Source: CAD feature listing. Evaluate the final solid. Frame: model axes, mm. A direction names the side the tool comes from. Give positions to 0.01 mm unless a question says otherwise; leave off trailing zeros. Order: outer loops, then holes, each group sorted by start corner. A loop starts at its lowest first (then second) coordinate and runs counter-clockwise, first axis right, second up. Notation, with made-up numbers: (37, 32) -> (94, 32) arc R18 ccw to (94, 61) -> close; hole circle Ø9 at (37, 4.5). An arc over 180 degrees is marked (long way). Answer in a Markdown table with one row per item.
```python
from build123d import *

# Parameters (mm, degrees)
BOSS_EXTRUDE6_DEPTH = 1
SKETCH7_R           = 1
CUT_EXTRUDE1_DEPTH  = 10


with BuildPart() as part:
    # Sketch3 → Boss-Extrude6 (new body)
    with BuildSketch(Plane(origin=(0, 0, 0), x_dir=(1, 0, 0), z_dir=(0, 1, 0))):
        with BuildLine():
            Line((24.032258065, -5), (26.532258065, -5))
            Line((26.532258065, -5), (26.532258065, 2))
            Line((26.532258065, 2), (41.532258065, 2))
            Line((41.532258065, 2), (41.532258065, 5))
            Line((41.532258065, 5), (26.532258065, 5))
            Line((26.532258065, 5), (-13.467741935, 5))
            Line((-13.467741935, 5), (-13.467741935, -5))
            Line((-13.467741935, -5), (9.032258065, -5))
            ThreePointArc((9.032258065, -5), (16.532258065, -12.5), (24.032258065, -5))
        make_face()
    extrude(amount=BOSS_EXTRUDE6_DEPTH)

    # Sketch7 → Cut-Extrude1 (cut)
    with BuildSketch(Plane.XZ):
        with Locations(Location((3.582258065, 2.38, 0), (0, 0, 270))):
            Circle(SKETCH7_R)
    extrude(amount=-CUT_EXTRUDE1_DEPTH, mode=Mode.SUBTRACT)


solid = part.part
```
(1) Section query A-A (z = 2.38). Return the cut outline in (x, y).
A:
| item | result |
|---|---|
| outline | (-13.47, 0) -> (2.58, 0) -> (2.58, 1) -> (-13.47, 1) -> close; (4.58, 0) -> (26.53, 0) -> (26.53, 1) -> (4.58, 1) -> close |
(2) Access query for faces 4 (the flat face through (33.9, 0.5, -2)), 5 (the flat face through (14, 0, 2)), 6 (the flat face through (-2.4, 0.5, 5)). Directions: +Z, -Z, +X, -X, +Y, -Y. A direction counts if a zero-diameter tool reaches every point of the face in a straight line with its end or side. Return the directions, or none.
A:
| item | result |
|---|---|
| face 4 | +Z, +X, +Y, -Y |
| face 5 | +Z, -Z, +X, -X, -Y |
| face 6 | +Z, -X, +Y, -Y |
(3) Section query C-C (x = -2). Return the cut outline in (y, z), plus the area to 3 significant figures.
A:
| item | result |
|---|---|
| outline | (0, -5) -> (1, -5) -> (1, 5) -> (0, 5) -> close |
| area | 10.0 mm^2 |
(4) Section query B-B (y = 0.25). Return the cut outline in (x, z), plus the area to 3 significant figures.
A:
| item | result |
|---|---|
| outline | (-13.47, -5) -> (41.53, -5) -> (41.53, -2) -> (26.53, -2) -> (26.53, 5) -> (24.03, 5) arc R7.5 ccw to (9.03, 5) -> (-13.47, 5) -> close; hole circle Ø2 at (3.58, 2.38) |
| area | 530 mm^2 |
(5) Ray query, probe 1 along X at (y, z) = (0.3, 2.38); probe 2 along Z at (x, y) = (-6.5, 0.95); probe 3 along Z at (x, y) = (37, 0.7). Return the intervals inside material, ascending.
A:
| item | result |
|---|---|
| probe 1 | x = -13.47 to 2.58, 4.58 to 26.53 |
| probe 2 | z = -5 to 5 |
| probe 3 | z = -5 to -2 |
(6) First-contact query: pin 1 Ø8 at (x, z) = (-1, 10) entering from +Y. Flat tip, straight axial feed; report the tip coordinate or a pass-through.
A:
| item | result |
|---|---|
| pin 1 | passes through |
(7) Pull-direction query (Z, two-part tool) for faces 1 (the cylindrical face through (4.425, 0.493, 1.842)), 2 (the flat face through (14.4, 0.5, -5)), 3 (the cylindrical face through (16.4, 0.5, 12.5)); classes: +Z half, -Z half, draft (parallel to the pull), parting line (faces both ways), or undercut.
A:
| item | result |
|---|---|
| face 1 | undercut |
| face 2 | -Z half |
| face 3 | +Z half |
(8) Section query D-D (z = -0.75). Return the cut outline in (x, y), plus the area to 3 significant figures.
A:
| item | result |
|---|---|
| outline | (-13.47, 0) -> (26.53, 0) -> (26.53, 1) -> (-13.47, 1) -> close |
| area | 40.0 mm^2 |
